```python
from build123d import *

# Parameters (mm, degrees)
SKETCH1_R           = 4.5
BOSS_EXTRUDE1_DEPTH = 1


with BuildPart() as part:
    # Sketch1 → Boss-Extrude1 (new body)
    with BuildSketch(Plane.XY):
        with BuildLine():
            Line((-61, 85.675899882), (-61, -85.675899882))
            ThreePointArc((-61, -85.675899882), (-60.121320344, -87.797220225), (-58, -88.675899882))
            Line((-58, -88.675899882), (58, -88.675899882))
            ThreePointArc((58, -88.675899882), (60.121320344, -87.797220225), (61, -85.675899882))
            Line((61, -85.675899882), (61, 85.675899882))
            ThreePointArc((61, 85.675899882), (60.221977932, 87.691542228), (58.291457286, 88.661708424))
            ThreePointArc((58.291457286, 88.661708424), (0, 91.5), (-58.291457286, 88.661708424))
            ThreePointArc((-58.291457286, 88.661708424), (-60.221977932, 87.691542228), (-61, 85.675899882))
        make_face()
        with Locations((-40, 74.5)):
            Circle(SKETCH1_R, mode=Mode.SUBTRACT)
        with Locations((-50, -9.5)):
            Circle(SKETCH1_R, mode=Mode.SUBTRACT)
        with Locations((-40, -74.5)):
            Circle(SKETCH1_R, mode=Mode.SUBTRACT)
        with Locations(Location((40, -74.5, 0), (0, 0, 180))):
            Circle(SKETCH1_R, mode=Mode.SUBTRACT)
        with Locations(Location((50, -9.5, 0), (0, 0, 180))):
            Circle(SKETCH1_R, mode=Mode.SUBTRACT)
        with Locations(Location((40, 74.5, 0), (0, 0, 180))):
            Circle(SKETCH1_R, mode=Mode.SUBTRACT)
        with BuildLine():
            Line((-41, -23.356406461), (-41, -51.434874811))
            ThreePointArc((-41, -51.434874811), (-39.113055385, -58.180243592), (-34, -62.967437405))
            ThreePointArc((-34, -62.967437405), (-31.68672135, -64.505531626), (-29.753049234, -66.5))
            ThreePointArc((-29.753049234, -66.5), (-25.206975594, -70.183321446), (-19.506098468, -71.5))
            Line((-19.506098468, -71.5), (19.506098468, -71.5))
            ThreePointArc((19.506098468, -71.5), (25.206975594, -70.183321446), (29.753049234, -66.5))
            ThreePointArc((29.753049234, -66.5), (31.68672135, -64.505531626), (34, -62.967437405))
            ThreePointArc((34, -62.967437405), (39.113055385, -58.180243592), (41, -51.434874811))
            Line((41, -51.434874811), (41, -23.356406461))
            ThreePointArc((41, -23.356406461), (40.489995997, -19.750855185), (39, -16.42820323))
            ThreePointArc((39, -16.42820323), (37, -9.5), (39, -2.57179677))
            ThreePointArc((39, -2.57179677), (40.489995997, 0.750855185), (41, 4.356406461))
            Line((41, 4.356406461), (41, 51.434874811))
            ThreePointArc((41, 51.434874811), (39.113055385, 58.180243592), (34, 62.967437405))
            ThreePointArc((34, 62.967437405), (31.68672135, 64.505531626), (29.753049234, 66.5))
            ThreePointArc((29.753049234, 66.5), (25.206975594, 70.183321446), (19.506098468, 71.5))
            Line((19.506098468, 71.5), (16.492422502, 71.5))
            ThreePointArc((16.492422502, 71.5), (10.818757356, 72.803439659), (6.28282762, 76.452380952))
            ThreePointArc((6.28282762, 76.452380952), (0, 79.5), (-6.28282762, 76.452380952))
            ThreePointArc((-6.28282762, 76.452380952), (-10.818757356, 72.803439659), (-16.492422502, 71.5))
            Line((-16.492422502, 71.5), (-19.506098468, 71.5))
            ThreePointArc((-19.506098468, 71.5), (-25.206975594, 70.183321446), (-29.753049234, 66.5))
            ThreePointArc((-29.753049234, 66.5), (-31.68672135, 64.505531626), (-34, 62.967437405))
            ThreePointArc((-34, 62.967437405), (-39.113055385, 58.180243592), (-41, 51.434874811))
            Line((-41, 51.434874811), (-41, 4.356406461))
            ThreePointArc((-41, 4.356406461), (-40.489995997, 0.750855185), (-39, -2.57179677))
            ThreePointArc((-39, -2.57179677), (-37, -9.5), (-39, -16.42820323))
            ThreePointArc((-39, -16.42820323), (-40.489995997, -19.750855185), (-41, -23.356406461))
        make_face(mode=Mode.SUBTRACT)
    extrude(amount=BOSS_EXTRUDE1_DEPTH)


solid = part.part
```
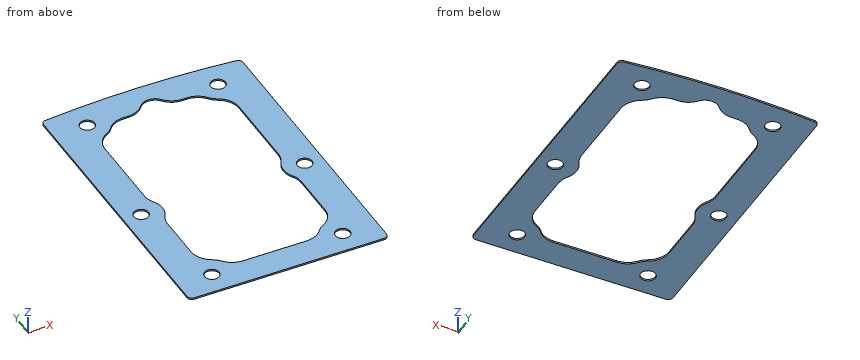
CAD build for the part. Positions are in the model's coordinates, mm. Round coordinates to 2 decimals unless told otherwise and drop trailing zeros. Loops run counter-clockwise (first coordinate to the right, second up) from the corner with the lowest first, then second, coordinate; pieces in that order, holes last. Notation, with made-up numbers: M 64.5,61 L 87.5,61 A23 cw 87.5,73 Z; hole C -9.5,-5.75 d9. An arc over 180 degrees is marked long. Return JSON: item names as keys, results as strings. Group by question number.
(1) Drop flat-ended pins along their axis: P1, Ø5.5, axis at x = 40, y = 74.5, coming from the -Z side; P2, Ø0.5, axis at x = 1, z = 0.5, coming from the +Y side. Give the stop position or say it passes through.
(2) Saw through at D-D, the plane z = 0.3. Give the number of separate pieces and of enclosed holes in the cut face, and give its area (3 significant figures).
(3) Saw through at A-A, the plane y = -9.5. List the corners of the cut face in (x, z), and give its area (3 significant figures).
(4) Wall check: probe 1 along X at (y, z) = (-49, 0.15); probe 2 along Y at (x, z) = (-40, 0.4); probe 3 along Y at (x, z) = (19.5, 0.75). Give the ranges that are in metal, low to high. Write a range as [from, to].
(5) Saw through at B-B, the plane y = 34. List the corners of the cut face in (x, z).
(6) Saw through at C-C, the plane x = -50. List the corners of the cut face in (y, z).
Answer list:
{
 "1": {"P1": "through", "P2": "y = 91.5"},
 "2": {"separate pieces": "1", "enclosed holes": "7", "area": "10,200 mm2"},
 "3": {"outline": "M -61,0 L -54.5,0 L -54.5,1 L -61,1 Z; M -45.5,0 L -37,0 L -37,1 L -45.5,1 Z; M 37,0 L 45.5,0 L 45.5,1 L 37,1 Z; M 54.5,0 L 61,0 L 61,1 L 54.5,1 Z", "area": "30.0 mm2"},
 "4": {"probe 1": "[-61, -41], [41, 61]", "probe 2": "[-88.68, -79], [-70, -56.43], [-18.36, -0.64], [56.43, 70], [79, 90.17]", "probe 3": "[-88.68, -71.5], [71.5, 91.18]"},
 "5": {"outline": "M -61,0 L -41,0 L -41,1 L -61,1 Z; M 41,0 L 61,0 L 61,1 L 41,1 Z"},
 "6": {"outline": "M -88.68,0 L -14,0 L -14,1 L -88.68,1 Z; M -5,0 L 89.41,0 L 89.41,1 L -5,1 Z"}
}
